```python
from build123d import *

# Parameters (mm, degrees)
ESQUISSE1_W        = 32
ESQUISSE1_H        = 32
BOSS_EXTRU_1_DEPTH = 35
ESQUISSE2_R        = 6.784029575
ESQUISSE2_R_2      = 3.677937746
BOSS_EXTRU_2_DEPTH = 15
ESQUISSE3_R        = 12.676726104
BOSS_EXTRU_3_DEPTH = 2


with BuildPart() as part:
    # Esquisse1 → Boss.-Extru.1 (new body)
    with BuildSketch(Plane.XY):
        Rectangle(ESQUISSE1_W, ESQUISSE1_H)
    extrude(amount=BOSS_EXTRU_1_DEPTH)

    # Esquisse2 → Boss.-Extru.2 (add)
    with BuildSketch(Plane.XY.offset(35)):
        Circle(ESQUISSE2_R)
        Circle(ESQUISSE2_R_2, mode=Mode.SUBTRACT)
    extrude(amount=BOSS_EXTRU_2_DEPTH)

    # Esquisse3 → Boss.-Extru.3 (add)
    with BuildSketch(Plane.XY.offset(35)):
        Circle(ESQUISSE3_R)
    extrude(amount=BOSS_EXTRU_3_DEPTH)


solid = part.part
```
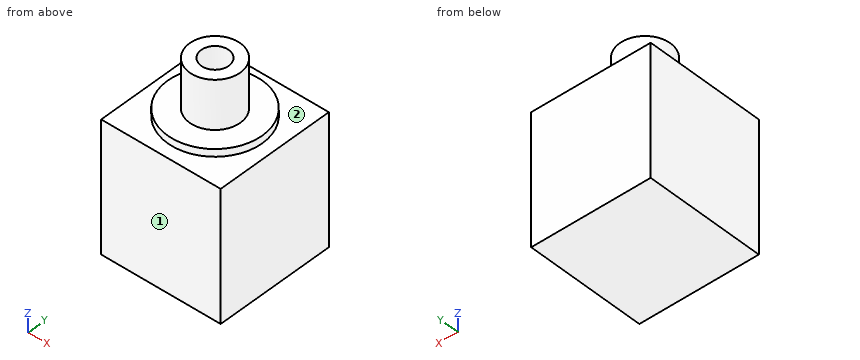
Work out the finished part from the listing and answer in its coordinate system (mm). Face numbers are marked on the shaded views. A direction names the side the tool comes from. Give positions to 0.01 mm unless a question says otherwise; leave off trailing zeros. Order: outer loops, then holes, each group sorted by start corner. A loop starts at its lowest first (then second) coordinate and runs counter-clockwise, first axis right, second up. Notation, with made-up numbers: (85.25, -24.5) -> (128.25, -24.5) arc R31 ccw to (128.25, 7.5) -> close; hole circle Ø8 at (53, -34.75). An arc over 180 degrees is marked (long way). Answer as CSV lines item,"result". Start each with the question number.
(1) Section D-D, the plane y = 10 is taken. Write down the section's boundary in (x, z), plus the area to 3 significant figures.
(2) Which of the six approach directions +Z, -Z, +X, -X, +Y, -Y give full straight-line access (tool end or side, diameter ignored) to the marked faces 1 and 2?
(3) Consider line 1 along X through (y, z) = (0, 46); line 2 along Z through (x, y) = (14, 2). Determine where each line is inside the solid, lowest interval first.
(4) Section C-C, the plane z = 41.5 is taken. Write down the section's boundary in (x, y), plus the area to 3 significant figures.
(5) Each of these flat-tipped pins is pushed along its axis until it touches: pin 1 Ø1.5 at (x, y) = (-1, 1) entering from +Z; pin 2 Ø12 at (x, z) = (5, 43.5) entering from -Y; pin 3 Ø6 at (y, z) = (-10, 42.5) entering from +X. Where does it stop, or does it pass through?
(6) Section A-A, the plane y = 0 is taken. Write down the section's boundary in (x, z), plus the area to 3 significant figures.
Entries:
1,outline,"(-16, 0) -> (16, 0) -> (16, 35) -> (7.79, 35) -> (7.79, 37) -> (-7.79, 37) -> (-7.79, 35) -> (-16, 35) -> close"
1,area,"1,150 mm²"
2,face 1,"+Z, -Z, +X, -X, -Y"
2,face 2,"+Z"
3,line 1,"-6.78 to -3.68, 3.68 to 6.78"
3,line 2,"0 to 35"
4,outline,"circle Ø13.57 at (0, 0); hole circle Ø7.36 at (0, 0)"
4,area,"102 mm²"
5,pin 1,"z = 37"
5,pin 2,"y = -6.78"
5,pin 3,"through"
6,outline,"(-16, 0) -> (16, 0) -> (16, 35) -> (12.68, 35) -> (12.68, 37) -> (6.78, 37) -> (6.78, 50) -> (3.68, 50) -> (3.68, 37) -> (-3.68, 37) -> (-3.68, 50) -> (-6.78, 50) -> (-6.78, 37) -> (-12.68, 37) -> (-12.68, 35) -> (-16, 35) -> close"
6,area,"1,250 mm²"
